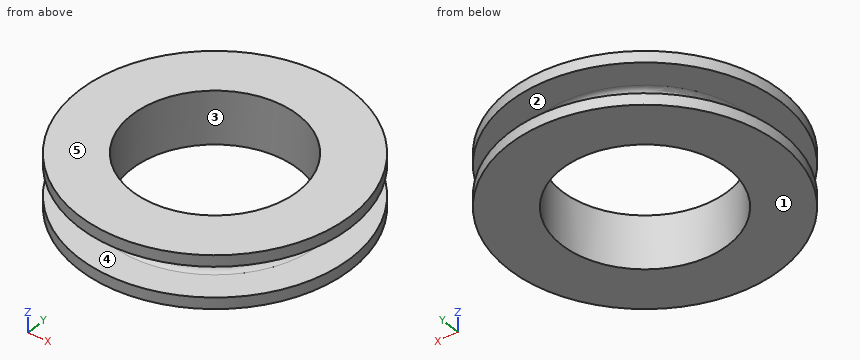
from build123d import *

# Parameters (mm, degrees)
F2_R = 1


with BuildPart() as f1:
    # F0 (on Front) → F1 (revolve)
    with BuildSketch(Plane.XZ):
        Polygon((18, 3.5), (11, 3.5), (11, 0), (11, -3.5), (18, -3.5), (18, -2), (13, -2), (13, 0), (13, 2), (18, 2), align=None)
    revolve(axis=Axis((0, 0, 1.75), (0, 0, 1)))

    # F2
    f2_edges = [f1.edges().sort_by_distance(p)[0] for p in [
        (-13, 0, -2),
        (13, 0, 0),
        (-13, 0, 2),
    ]]
    fillet(f2_edges, radius=F2_R)


solid = f1.part
Read the model definition and answer for the solid it produces. Units are mm, in the model's axes. Face numbers are marked on the shaded views. A direction names the side the tool comes from. Round coordinates to 2 decimals unless told otherwise and drop trailing zeros. Write each loop counter-clockwise with the first axis right and the second up, starting at its lowest first coordinate (ties: lowest second). Pieces come first, ordered by that corner, then holes.
1. Determine the mould class of the marked faces 1, 2 and 3 for opening direction Z: pulls with the +Z half, pulls with the -Z half, needs draft (parallel to the pull), parting line crosses it, or undercut.
2. The part is cut by section A-A, the plane x = 0. Determine the outline of the cut face in (y, z), then the cut area to 3 significant figures.
3. Straight lines are drawn through the part: L1, parallel to Z at x = 12.5, y = -12.5; L2, parallel to Y at x = 0, z = -1; L3, parallel to Y at x = 2.5, z = -0.25. For each, find the intervals that lie inside material, in ascending order.
4. Which of the six approach directions +Z, -Z, +X, -X, +Y, -Y give full straight-line access (tool end or side, diameter ignored) to the marked faces 4 and 5?
5. Given pin 1 Ø1.5 at (x, z) = (-14, 1.5) entering from -Y; pin 2 Ø3 at (x, z) = (10, -1) entering from -Y; pin 3 Ø4 at (x, z) = (11.5, -1) entering from -Y, each flat-ended and moving along its own axis, determine where each tip first touches the part or whether it passes through.
6. The part is cut by section C-C, the plane z = 3. Determine the outline of the cut face in (x, y), then the cut area to 3 significant figures.
Values:
1. face 1: pulls with the -Z half
1. face 2: undercut
1. face 3: needs draft
2. outline: (-18, -3.5) - (-11, -3.5) - (-11, 3.5) - (-18, 3.5) - (-18, 2) - (-14, 2) arc R1 cw to (-13, 1) - (-13, -1) arc R1 cw to (-14, -2) - (-18, -2) - close; (11, -3.5) - (18, -3.5) - (18, -2) - (14, -2) arc R1 cw to (13, -1) - (13, 1) arc R1 cw to (14, 2) - (18, 2) - (18, 3.5) - (11, 3.5) - close
2. area: 58.9 mm2
3. L1: z = -3.5 to -2, 2 to 3.5
3. L2: y = -13 to -11, 11 to 13
3. L3: y = -12.76 to -10.71, 10.71 to 12.76
4. face 4: none
4. face 5: +Z, +X, -X, +Y, -Y
5. pin 1: stops at y = -11.97
5. pin 2: stops at y = -15.66
5. pin 3: stops at y = -15.12
6. outline: circle Ø36 at (0, 0); hole circle Ø22 at (0, 0)
6. area: 638 mm2
